Input: part model. Units: mm. Frame: model coordinates. Face numbers are marked on the shaded views. A direction names the side the tool comes from. Give positions to 0.01 mm unless a question says otherwise; leave off trailing zeros. Order: outer loops, then holes, each group sorted by start corner. A loop starts at its lowest first (then second) coordinate and runs counter-clockwise, first axis right, second up. Notation, with made-up numbers: (44, -20.75) - (54, -20.75) arc R28 cw to (54, 1.25) - close; hole circle Ø9 at (7, 41.5). An arc over 180 degrees is marked (long way). Answer in a Markdown table with one row per item. Add a question column.
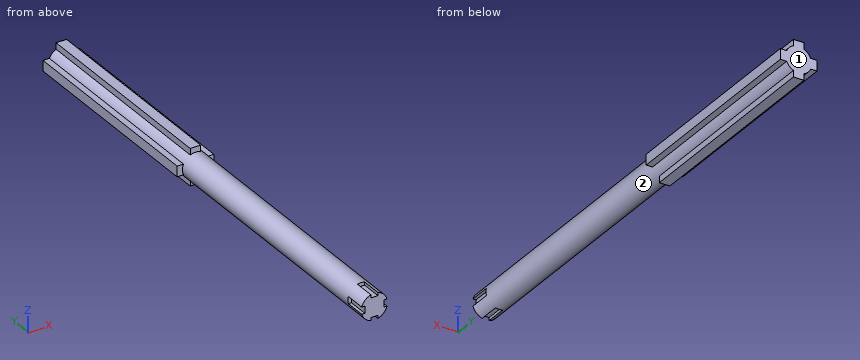
Autodesk Inventor part; units mm, degrees
ref_plane "YZ Plane" through (0, 0, 0) normal (1, 0, 0) x (0, 1, 0)
ref_plane "XZ Plane" through (0, 0, 0) normal (0, 1, 0) x (-1, 0, 0)
ref_plane "XY Plane" through (0, 0, 0) normal (0, 0, 1) x (1, 0, 0)
sketch "Sketch7" plane through (0, 0, 0) normal (0, 1, 0) x (-1, 0, 0)
  circle A0 centre (0, 0) radius 3.75
  dimension "d71" = 7.5
extrude "Extrusion7" add sketch "Sketch7" along normal blind 130
sketch "Sketch8" plane through (0, 130, 0) normal (0, 1, 0) x (1, 0, 0)
  line L0 (-5.25, -1.5) -> (-2.25, -1.5)
  line L1 (-2.25, -1.5) -> (-2.25, 1.5)
  line L2 (-2.25, 1.5) -> (-5.25, 1.5)
  line L3 (-5.25, 1.5) -> (-5.25, -1.5)
  circle A0 centre (0, 0) radius 3.75
  line L4 (-5.25, -1.5) -> (-2.25, 1.5) construction
  line L5 (-2.25, -1.5) -> (-5.25, 1.5) construction
  line L6 (1.5, 2.25) -> (-1.5, 2.25)
  line L7 (-1.5, 2.25) -> (-1.5, 5.25)
  line L8 (-1.5, 5.25) -> (1.5, 5.25)
  line L9 (1.5, 5.25) -> (1.5, 2.25)
  line L10 (1.5, 2.25) -> (-1.5, 5.25) construction
  line L11 (-1.5, 2.25) -> (1.5, 5.25) construction
  line L12 (2.25, -1.5) -> (5.25, -1.5)
  line L13 (5.25, -1.5) -> (5.25, 1.5)
  line L14 (5.25, 1.5) -> (2.25, 1.5)
  line L15 (2.25, 1.5) -> (2.25, -1.5)
  line L16 (2.25, -1.5) -> (5.25, 1.5) construction
  line L17 (5.25, -1.5) -> (2.25, 1.5) construction
  line L18 (-1.5, -5.25) -> (1.5, -5.25)
  line L19 (1.5, -5.25) -> (1.5, -2.25)
  line L20 (1.5, -2.25) -> (-1.5, -2.25)
  line L21 (-1.5, -2.25) -> (-1.5, -5.25)
  line L22 (-1.5, -5.25) -> (1.5, -2.25) construction
  line L23 (1.5, -5.25) -> (-1.5, -2.25) construction
  point P0 (-3.75, 0)
  point P1 (0, 3.75)
  point P2 (3.75, 0)
  point P3 (0, -3.75)
  point P4 (3.4369, 1.5)
  point P5 (3.4369, -1.5)
  point P6 (-1.5, 3.4369)
  point P7 (1.5, 3.4369)
  point P8 (-3.4369, -1.5)
  point P9 (-3.4369, 1.5)
  point P10 (1.5, -3.4369)
  point P11 (-1.5, -3.4369)
  dimension "d74" = 3
  dimension "d75" = 3
  dimension "d76" = 3
  dimension "d77" = 3
  dimension "d78" = 3
  dimension "d79" = 3
  dimension "d80" = 3
  dimension "d81" = 3
extrude "Extrusion8" add sketch "Sketch8" along normal blind 10 and the other way blind 50
sketch "Sketch9" plane through (0, 0, 0) normal (0, -1, 0) x (1, 0, 0)
  line L0 (4.75, 1) -> (2.75, 1)
  line L1 (2.75, 1) -> (2.75, -1)
  line L2 (2.75, -1) -> (4.75, -1)
  line L3 (4.75, -1) -> (4.75, 1)
  arc A0 (3.4369, -1.5) -> (3.4369, 1.5) centre (0, 0) ccw
  line L4 (4.75, 1) -> (2.75, -1) construction
  line L5 (2.75, 1) -> (4.75, -1) construction
  line L6 (1, -2.75) -> (-1, -2.75)
  line L7 (-1, -2.75) -> (-1, -4.75)
  line L8 (-1, -4.75) -> (1, -4.75)
  line L9 (1, -4.75) -> (1, -2.75)
  arc A1 (-1.5, -3.4369) -> (1.5, -3.4369) centre (0, 0) ccw
  line L10 (1, -2.75) -> (-1, -4.75) construction
  line L11 (-1, -2.75) -> (1, -4.75) construction
  line L12 (-2.75, 1) -> (-4.75, 1)
  line L13 (-4.75, 1) -> (-4.75, -1)
  line L14 (-4.75, -1) -> (-2.75, -1)
  line L15 (-2.75, -1) -> (-2.75, 1)
  arc A2 (-3.4369, 1.5) -> (-3.4369, -1.5) centre (0, 0) ccw
  line L16 (-2.75, 1) -> (-4.75, -1) construction
  line L17 (-4.75, 1) -> (-2.75, -1) construction
  line L18 (1, 4.75) -> (-1, 4.75)
  line L19 (-1, 4.75) -> (-1, 2.75)
  line L20 (-1, 2.75) -> (1, 2.75)
  line L21 (1, 2.75) -> (1, 4.75)
  line L22 (1, 4.75) -> (-1, 2.75) construction
  line L23 (-1, 4.75) -> (1, 2.75) construction
  point P0 (3.75, 0)
  point P1 (0, -3.75)
  point P2 (-3.75, 0)
  point P3 (0, 3.75)
  point P4 (-3.6142, 1)
  point P5 (-3.6142, -1)
  point P6 (-1, -3.6142)
  point P7 (1, -3.6142)
  point P8 (3.6142, -1)
  point P9 (3.6142, 1)
  dimension "d86" = 2
  dimension "d87" = 2
  dimension "d88" = 2
  dimension "d89" = 2
  dimension "d90" = 2
  dimension "d91" = 2
  dimension "d92" = 2
  dimension "d93" = 2
extrude "Extrusion9" cut sketch "Sketch9" against normal blind 6 contours A0 L2 L1 L0 | L9 A1 L7 L6 | L15 L14 A2 L12 | L21 L20 L19 L18
properties part number "Lower Arm"
Q1. Access query for the marked faces 1 and 2. Directions: +Z, -Z, +X, -X, +Y, -Y. A direction counts if a zero-diameter tool reaches every point of the face in a straight line with its end or side. Return the directions, or none.
Q2. Line query: probe 1 along X at (y, z) = (132.5, -3.5); probe 2 along X at (y, z) = (78, 0.25). Output: solid intervals per line, ascending.
Q3. Section A-A, the plane y = 10. Return loops of the section in (x, z), then the cut area to 3 significant figures.
Q4. Contact query for flat-ended pins moving along their axis: P1, Ø2, axis at x = 4.5, y = 96, coming from the -Z side; P2, Ø0.9, axis at x = -4.5, z = 0.5, coming from the -Y side; P3, Ø2, axis at y = 49.5, z = -0.5, coming from the -X side. Output: stop coordinate, or through.
Computed:
| question | item | result |
|---|---|---|
| 1 | face 1 | +Z, -Z, +X, -X, +Y |
| 1 | face 2 | -Y |
| 2 | probe 1 | x = -1.5 to 1.5 |
| 2 | probe 2 | x = -3.74 to 3.74 |
| 3 | outline | circle Ø7.5 at (0, 0) |
| 3 | area | 44.2 mm^2 |
| 4 | P1 | stops at z = -1.5 |
| 4 | P2 | stops at y = 80 |
| 4 | P3 | stops at x = -3.75 |
